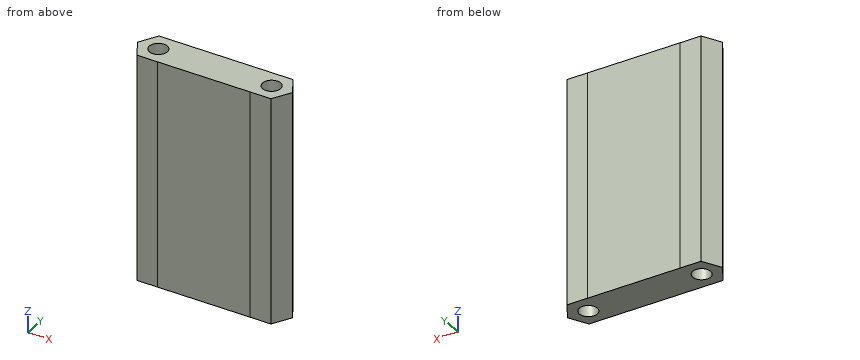
Autodesk Inventor part; units mm, degrees
sketch "Sketch2" plane through (0, 0, 0) normal (0, 0, 1) x (1, 0, 0)
  line L0 (0, 2.8582) -> (0, -2.8582) construction
  line L1 (-5.7775, 0) -> (5.7775, 0) construction
  line L2 (0, 0) -> (4, 0)
  line L3 (4, 0) -> (-4, 0)
  circle A0 centre (0, 0) radius 4
  line L4 (0, 0) -> (-2, 3.4641)
  line L5 (0, 0) -> (4, 0) construction
  line L6 (0, 0) -> (2, 3.4641)
  line L7 (0, 0) -> (4, 0) construction
  line L8 (0, 0) -> (4, 0)
  line L9 (0, 0) -> (2, -3.4641)
  line L10 (0, 0) -> (-2, -3.4641)
  line L11 (-2, 3.4641) -> (2, 3.4641)
  line L12 (2, 3.4641) -> (4, 0)
  line L13 (4, 0) -> (2, -3.4641)
  line L14 (2, -3.4641) -> (-2, -3.4641)
  line L15 (-2, -3.4641) -> (-4, 0)
  line L16 (-4, 0) -> (-2, 3.4641)
  dimension "d3" = 4
  dimension "d2" = 8
  dimension "d1" = 120
  dimension "d0" = 60
extrude "Extrusion1" add sketch "Sketch2" along normal blind 43.5 contours L6 L12 L2 | L10 L15 L3 | L3 L16 L4 | L4 L11 L6 | L2 L13 L9 | L9 L14 L10
sketch "Sketch3" plane through (0, 0, 43.5) normal (0, 0, 1) x (1, 0, 0)
  point P0 (0, 0)
  point P1 (0, 0)
hole "Hole1" at (0, 0, 43.5) direction (0, 0, -1) diameter 3.4587 depth 44
sketch "Sketch5" plane through (0, 0, 43.5) normal (0, 0, 1) x (1, 0, 0)
  line L0 (0, 0) -> (21.751, 0)
  line L1 (21.751, 0) -> (25.751, 0)
  line L2 (21.751, 0) -> (21.751, 3.464)
  line L3 (21.751, 3.464) -> (23.751, 3.464)
  line L4 (23.751, 3.464) -> (25.751, 0)
  line L5 (21.751, 3.464) -> (19.751, 3.464)
  line L6 (21.751, 0) -> (17.751, 0)
  line L7 (17.751, 0) -> (19.751, 3.464)
  line L8 (21.751, 0) -> (21.751, -3.464)
  line L9 (21.751, -3.464) -> (23.751, -3.464)
  line L10 (23.751, -3.464) -> (25.751, 0)
  line L11 (21.751, -3.464) -> (19.751, -3.464)
  line L12 (19.751, -3.464) -> (17.751, 0)
  line L13 (2, 3.4641) -> (-2, 3.4641)
  line L14 (0, 3.4641) -> (21.751, 3.464)
  line L15 (21.751, -3.464) -> (0, -3.4641)
  line L16 (-2, -3.4641) -> (2, -3.4641)
  line L17 (4, 0) -> (2, 3.4641)
  line L18 (0, 3.4641) -> (4, 0)
  line L19 (4, 0) -> (0, -3.4641)
  point P0 (2, 3.4641)
  point P1 (63.19, -3.464)
  point P2 (63.19, 3.464)
  dimension "d29" = 21.751
  dimension "d28" = 4
  dimension "d27" = 3.464
  dimension "d26" = 2
  dimension "d25" = 2
  dimension "d24" = 4
  dimension "d23" = 3.464
  dimension "d22" = 2
  dimension "d21" = 2
extrude "Extrusion2" add sketch "Sketch5" against normal blind 43.5
sketch "Sketch6" plane through (0, 0, 43.5) normal (0, 0, 1) x (1, 0, 0)
  line L0 (0, 0) -> (21.751, 0)
  dimension "d34" = 21.751
hole "Hole3" at (21.751, 0, 43.5) direction (0, 0, -1) diameter 3.4587 depth 44
properties part number "Steunstuk kort" material "S235"
Read the model definition and answer for the solid it produces. Units are mm, in the model's axes. Round coordinates to 2 decimals unless told otherwise and drop trailing zeros. Write each loop counter-clockwise with the first axis right and the second up, starting at its lowest first coordinate (ties: lowest second). Pieces come first, ordered by that corner, then holes. Notation, with made-up numbers: (35, 17.5) - (49, 17.5) arc R26 ccw to (49, 44.5) - close; hole circle Ø2 at (4.5, 47). An arc over 180 degrees is marked (long way). One line per question, with ' | ' between items. Start each with the question number.
1. Find the intervals of material crossed by probe 1 along X at (y, z) = (0, 21); probe 2 along Y at (x, z) = (0, 25.5); probe 3 along X at (y, z) = (0.75, 4.5), in increasing order. Write a range as [from, to].
2. Each of these flat-tipped pins is pushed along its axis until it touches: pin 1 (1 mm diameter, centred on y = 2, z = 38.5, fed in from +X); pin 2 (4 mm diameter, centred on y = 0, z = 15, fed in from -X). Where does it stop, or does it pass through?
3. Section A-A (x = 0) is taken. Determine the outline of the cut face in (y, z), and give its area (3 significant figures).
4. Section C-C (y = -2.25) is taken. Determine the outline of the cut face in (x, z).
5. Section B-B (z = 10) is taken. Determine the outline of the cut face in (x, y).
Filled in:
1) probe 1: [-4, -1.73], [1.73, 20.02], [23.48, 25.75] | probe 2: [-3.46, -1.73], [1.73, 3.46] | probe 3: [-3.57, -1.56], [1.56, 20.19], [23.31, 25.32]
2) pin 1: x = 24.88 | pin 2: x = -4
3) outline: (-3.46, 0) - (-1.73, 0) - (-1.73, 43.5) - (-3.46, 43.5) - close; (1.73, 0) - (3.46, 0) - (3.46, 43.5) - (1.73, 43.5) - close | area: 151 mm²
4) outline: (-2.7, 0) - (24.45, 0) - (24.45, 43.5) - (-2.7, 43.5) - close
5) outline: (-4, 0) - (-2, -3.46) - (2, -3.46) - (19.75, -3.46) - (23.75, -3.46) - (25.75, 0) - (23.75, 3.46) - (19.75, 3.46) - (2, 3.46) - (-2, 3.46) - close; hole circle Ø3.46 at (0, 0); hole circle Ø3.46 at (21.75, 0)
